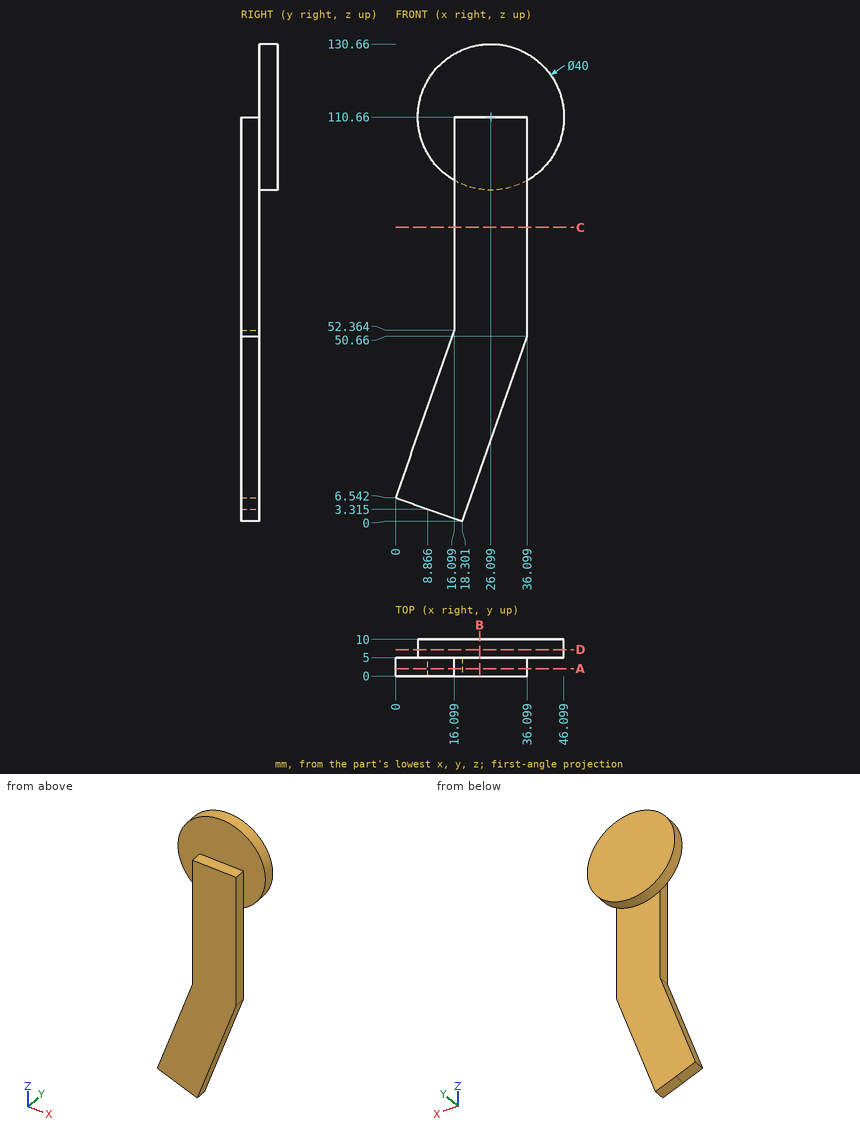
Verification items for this drawing (mm, ordinates from the low corner). Give positions to 0.01 mm unless a question says otherwise; leave off trailing zeros. Write each loop counter-clockwise with the first axis right and the second up, starting at its lowest first coordinate (ties: lowest second). Pieces come first, ordered by that corner, then holes.
1) Thickness scan on line 1 (Y direction, x = 22.5, z = 113); line 2 (Y direction, x = 26, z = 41); line 3 (X direction, y = 1.5, z = 64.5). Record the ranges inside material, lowest first.
Values follow:
line 1: y = 5 to 10
line 2: y = 0 to 5
line 3: x = 16.1 to 36.1
2) Cross-section at B-B (x = 23). Record the boundary of the cut face in (y, z) (1 decimal).
Values follow:
outline: (0, 13.4) - (5, 13.4) - (5, 90.9) - (10, 90.9) - (10, 130.4) - (5, 130.4) - (5, 110.7) - (0, 110.7) - close
3) Cross-section at D-D (y = 7.25). Record the boundary of the cut face in (x, z).
Values follow:
outline: circle Ø40 at (26.1, 110.66)
4) Go/stop test with flat-tipped pins: pin 1 Ø1.5 at (y, z) = (6.5, 16) entering from +X; pin 2 Ø1.5 at (y, z) = (2.5, 67.5) entering from -X; pin 3 Ø2 at (x, y) = (24.5, 5) entering from +Z; pin 4 Ø6 at (x, y) = (23, 5.5) entering from +Z. Record where each tip stops, or that it passes through.
Values follow:
pin 1: passes through
pin 2: stops at x = 16.1
pin 3: stops at z = 130.65
pin 4: stops at z = 130.66
5) Cross-section at A-A (y = 2). Record the boundary of the cut face in (x, z) (1 decimal).
Values follow:
outline: (0, 6.5) - (8.9, 3.3) - (18.3, 0) - (36.1, 50.7) - (36.1, 110.7) - (16.1, 110.7) - (16.1, 52.4) - close
6) Cross-section at C-C (z = 80.5). Record the boundary of the cut face in (x, y).
Values follow:
outline: (16.1, 0) - (36.1, 0) - (36.1, 5) - (16.1, 5) - close
